from build123d import *

# Parameters (mm, degrees)
F1_DEPTH = 8
F2_R     = 1.9
F2_R_2   = 1.25
F3_DEPTH = 25
F4_W     = 4
F4_H     = 2.3
F5_DEPTH = 25
F7_DEPTH = 3


with BuildPart() as f1:
    # F0 (on Front) → F1 (new body)
    with BuildSketch(Plane.XZ):
        with BuildLine():
            ThreePointArc((0, 4), (1.171573, 1.171573), (4, 0))
            Line((4, 0), (28, 0))
            ThreePointArc((28, 0), (30.828427, 1.171573), (32, 4))
            ThreePointArc((32, 4), (30.828427, 6.828427), (28, 8))
            Line((28, 8), (4, 8))
            ThreePointArc((4, 8), (1.171573, 6.828427), (0, 4))
        make_face()
    extrude(amount=-F1_DEPTH)

    # F2 (on face) → F3 (cut)
    with BuildSketch(Plane.XZ):
        with Locations((4, 4)):
            Circle(F2_R)
        with Locations((11.3, 4)):
            Circle(F2_R_2)
        with Locations((28.4, 4)):
            Circle(F2_R_2)
    extrude(amount=-F3_DEPTH, mode=Mode.SUBTRACT)

    # F4 (on face) → F5 (cut)
    with BuildSketch(Plane.XY.offset(8)):
        Polygon((4, 8), (4, 5.7), (8, 5.7), (24.5, 8), align=None)
        with Locations((2, 6.85)):
            Rectangle(F4_W, F4_H)
    extrude(amount=-F5_DEPTH, mode=Mode.SUBTRACT)

    # F6 (on face) → F7 (cut)
    with BuildSketch(Plane.XZ):
        with BuildLine():
            ThreePointArc((11.3, 7), (14.3, 4), (11.3, 1))
            Line((11.3, 1), (28.4, 1))
            ThreePointArc((28.4, 1), (25.4, 4), (28.4, 7))
            Line((28.4, 7), (11.3, 7))
        make_face()
    extrude(amount=-F7_DEPTH, mode=Mode.SUBTRACT)


solid = f1.part
The model under review builds one solid part; all positions refer to its coordinate system, in mm. A direction names the side the tool comes from. Round coordinates to 2 decimals unless told otherwise and drop trailing zeros. Write each loop counter-clockwise with the first axis right and the second up, starting at its lowest first coordinate (ties: lowest second). Pieces come first, ordered by that corner, then holes. Notation, with made-up numbers: M -38,57.25 L 21,57.25 A19 ccw 21,75.25 Z; hole C 47,-19.5 d9. An arc over 180 degrees is marked long. Use a Markdown table: item, result. Add a question column.
Q1. We need section A-A, the plane x = 26. State the section outline as (y, z) points, plus the area to 3 significant figures.
Q2. To check wall thickness, follow line 1 (Z direction, x = 4, y = 2.75); line 2 (Z direction, x = 21.5, y = 1.75); line 3 (Y direction, x = 7.5, z = 5). State the ranges of each line that lie inside material, in increasing order.
Q3. The part is to be moulded in two halves that separate along Z. For faces 1 (the face through (16, 3, 8)), 2 (the face through (14.3, 1.5, 4.1)), 3 (the face through (12, 0, 6)), say which applies: pulls with the +Z half, pulls with the -Z half, needs draft (parallel to the pull), parting line crosses it, or undercut.
Q4. We need section B-B, the plane y = 7.5. State the section outline as (x, z) points.
Q5. We need section C-C, the plane z = 6.5. State the section outline as (x, y) points, plus the area to 3 significant figures.
Q6. Insertion check: pin 1 (1.5 mm diameter, centred on y = 3, z = 1, fed in from +X); pin 2 (1 mm diameter, centred on y = 5, z = 3, fed in from +X); pin 3 (1.5 mm diameter, centred on y = 4, z = 2.5, fed in from -X); pin 4 (4 mm diameter, centred on x = 11.3, z = 4, fed in from -Y). Each pin has a flat end and moves straight along its axis. Give the tip position at first contact, or say it passes through.
Q7. Machinability: for faces 4 (the face through (20, 3, 4)), 5 (the face through (6, 5.7, 3)), 6 (the face through (2.6, 2.81, 5.284)), which of the approach directions +Z, -Z, +X, -X, +Y, -Y give a long, thin tool a straight path to every point of the face, cutting with its end or side? Answer none if there is none.
Q8. We need section D-D, the plane x = 12. State the section outline as (y, z) points, plus the area to 3 significant figures.
Findings below:
| question | item | result |
|---|---|---|
| 1 | outline | M 0,0 L 8,0 L 8,8 L 0,8 L 0,7 L 3,7 L 3,5.8 L 0,5.8 L 0,2.2 L 3,2.2 L 3,1 L 0,1 Z |
| 1 | area | 56.8 mm² |
| 2 | line 1 | z = 0 to 2.1, 5.9 to 8 |
| 2 | line 2 | z = 0 to 1, 7 to 8 |
| 2 | line 3 | y = 0 to 5.7 |
| 3 | face 1 | pulls with the +Z half |
| 3 | face 2 | undercut |
| 3 | face 3 | needs draft |
| 4 | outline | M 20.91,0 L 28,0 A4 ccw 28,8 L 20.91,8 Z; hole C 28.4,4 d2.5 |
| 5 | outline | M 0.88,0 L 12.96,0 L 12.96,3 L 26.74,3 L 26.74,0 L 31.12,0 L 31.12,8 L 24.5,8 L 8,5.7 L 0.88,5.7 Z |
| 5 | area | 165 mm² |
| 6 | pin 1 | stops at x = 31.31 |
| 6 | pin 2 | stops at x = 31.97 |
| 6 | pin 3 | stops at x = 0.07 |
| 6 | pin 4 | stops at y = 0 |
| 7 | face 4 | -Y |
| 7 | face 5 | +Z, -Z, -X, +Y |
| 7 | face 6 | +Y, -Y |
| 8 | outline | M 0,0 L 6.26,0 L 6.26,2.96 L 0,2.96 L 0,1.08 L 3,1.08 L 3,1 L 0,1 Z; M 0,5.04 L 6.26,5.04 L 6.26,8 L 0,8 L 0,7 L 3,7 L 3,6.92 L 0,6.92 Z |
| 8 | area | 36.6 mm² |
